Design review of the part built by this model. Coordinates are the model's own, in mm. Round coordinates to 2 decimals unless told otherwise and drop trailing zeros. Order: outer loops, then holes, each group sorted by start corner. A loop starts at its lowest first (then second) coordinate and runs counter-clockwise, first axis right, second up. Notation, with made-up numbers: (21.5, 3.5) - (50.5, 3.5) arc R26 cw to (50.5, 19.5) - close; hole circle Ø1 at (-17, 77.5). An arc over 180 degrees is marked (long way). Use CSV: the item, a comma, the result in double quotes.
from build123d import *

# Parameters (mm, degrees)
SKETCH1_W           = 63.2
SKETCH1_H           = 43.1
BOSS_EXTRUDE1_DEPTH = 1
CUT_EXTRUDE1_REACH  = 78.504
SKETCH2_R           = 1.25
CUT_EXTRUDE2_REACH  = 78.504
SKETCH3_R           = 0.4
CUT_EXTRUDE18_REACH = 78.504
SKETCH25_R          = 1.663368104


with BuildPart() as part:
    # Sketch1 → Boss-Extrude1 (new body)
    with BuildSketch(Plane(origin=(0, 0, 0), x_dir=(1, 0, 0), z_dir=(0, 1, 0))):
        with Locations((31.6, 21.55)):
            Rectangle(SKETCH1_W, SKETCH1_H)
    extrude(amount=BOSS_EXTRUDE1_DEPTH)

    # Sketch2 → Cut-Extrude1 (cut, up to next)
    with BuildSketch(Plane(origin=(0, 1, 0), x_dir=(1, 0, 0), z_dir=(0, 1, 0)), mode=Mode.PRIVATE) as cut_extrude1_sk1:
        with Locations(Location((3.5, 40.1, 0), (0, 0, 270))):
            Circle(SKETCH2_R)
    cut_extrude1_tool1 = extrude(cut_extrude1_sk1.sketch, amount=-CUT_EXTRUDE1_REACH, mode=Mode.PRIVATE) & part.part
    # Sketch2 → Cut-Extrude1 (cut, up to next)
    with BuildSketch(Plane(origin=(0, 1, 0), x_dir=(1, 0, 0), z_dir=(0, 1, 0)), mode=Mode.PRIVATE) as cut_extrude1_sk2:
        with Locations(Location((59.7, 40.1, 0), (0, 0, 270))):
            Circle(SKETCH2_R)
    cut_extrude1_tool2 = extrude(cut_extrude1_sk2.sketch, amount=-CUT_EXTRUDE1_REACH, mode=Mode.PRIVATE) & part.part
    # Sketch2 → Cut-Extrude1 (cut, up to next)
    with BuildSketch(Plane(origin=(0, 1, 0), x_dir=(1, 0, 0), z_dir=(0, 1, 0)), mode=Mode.PRIVATE) as cut_extrude1_sk3:
        with Locations(Location((59.7, 3, 0), (0, 0, 270))):
            Circle(SKETCH2_R)
    cut_extrude1_tool3 = extrude(cut_extrude1_sk3.sketch, amount=-CUT_EXTRUDE1_REACH, mode=Mode.PRIVATE) & part.part
    # Sketch2 → Cut-Extrude1 (cut, up to next)
    with BuildSketch(Plane(origin=(0, 1, 0), x_dir=(1, 0, 0), z_dir=(0, 1, 0)), mode=Mode.PRIVATE) as cut_extrude1_sk4:
        with Locations(Location((3.5, 3, 0), (0, 0, 270))):
            Circle(SKETCH2_R)
    cut_extrude1_tool4 = extrude(cut_extrude1_sk4.sketch, amount=-CUT_EXTRUDE1_REACH, mode=Mode.PRIVATE) & part.part
    add(cut_extrude1_tool1.solids().sort_by_distance((3.5, 1, -40.1))[0], mode=Mode.SUBTRACT)
    add(cut_extrude1_tool2.solids().sort_by_distance((59.7, 1, -40.1))[0], mode=Mode.SUBTRACT)
    add(cut_extrude1_tool3.solids().sort_by_distance((59.7, 1, -3))[0], mode=Mode.SUBTRACT)
    add(cut_extrude1_tool4.solids().sort_by_distance((3.5, 1, -3))[0], mode=Mode.SUBTRACT)

    # Sketch3 → Cut-Extrude2 (cut, up to next)
    with BuildSketch(Plane(origin=(0, 1, 0), x_dir=(1, 0, 0), z_dir=(0, 1, 0)), mode=Mode.PRIVATE) as cut_extrude2_sk1:
        with Locations(Location((7.47, 2.5, 0), (0, 0, 270))):
            Circle(SKETCH3_R)
    cut_extrude2_tool1 = extrude(cut_extrude2_sk1.sketch, amount=-CUT_EXTRUDE2_REACH, mode=Mode.PRIVATE) & part.part
    # Sketch3 → Cut-Extrude2 (cut, up to next)
    with BuildSketch(Plane(origin=(0, 1, 0), x_dir=(1, 0, 0), z_dir=(0, 1, 0)), mode=Mode.PRIVATE) as cut_extrude2_sk2:
        with Locations(Location((10.01, 2.5, 0), (0, 0, 270))):
            Circle(SKETCH3_R)
    cut_extrude2_tool2 = extrude(cut_extrude2_sk2.sketch, amount=-CUT_EXTRUDE2_REACH, mode=Mode.PRIVATE) & part.part
    # Sketch3 → Cut-Extrude2 (cut, up to next)
    with BuildSketch(Plane(origin=(0, 1, 0), x_dir=(1, 0, 0), z_dir=(0, 1, 0)), mode=Mode.PRIVATE) as cut_extrude2_sk3:
        with Locations(Location((12.55, 2.5, 0), (0, 0, 270))):
            Circle(SKETCH3_R)
    cut_extrude2_tool3 = extrude(cut_extrude2_sk3.sketch, amount=-CUT_EXTRUDE2_REACH, mode=Mode.PRIVATE) & part.part
    # Sketch3 → Cut-Extrude2 (cut, up to next)
    with BuildSketch(Plane(origin=(0, 1, 0), x_dir=(1, 0, 0), z_dir=(0, 1, 0)), mode=Mode.PRIVATE) as cut_extrude2_sk4:
        with Locations(Location((15.09, 2.5, 0), (0, 0, 270))):
            Circle(SKETCH3_R)
    cut_extrude2_tool4 = extrude(cut_extrude2_sk4.sketch, amount=-CUT_EXTRUDE2_REACH, mode=Mode.PRIVATE) & part.part
    # Sketch3 → Cut-Extrude2 (cut, up to next)
    with BuildSketch(Plane(origin=(0, 1, 0), x_dir=(1, 0, 0), z_dir=(0, 1, 0)), mode=Mode.PRIVATE) as cut_extrude2_sk5:
        with Locations(Location((17.63, 2.5, 0), (0, 0, 270))):
            Circle(SKETCH3_R)
    cut_extrude2_tool5 = extrude(cut_extrude2_sk5.sketch, amount=-CUT_EXTRUDE2_REACH, mode=Mode.PRIVATE) & part.part
    # Sketch3 → Cut-Extrude2 (cut, up to next)
    with BuildSketch(Plane(origin=(0, 1, 0), x_dir=(1, 0, 0), z_dir=(0, 1, 0)), mode=Mode.PRIVATE) as cut_extrude2_sk6:
        with Locations(Location((20.17, 2.5, 0), (0, 0, 270))):
            Circle(SKETCH3_R)
    cut_extrude2_tool6 = extrude(cut_extrude2_sk6.sketch, amount=-CUT_EXTRUDE2_REACH, mode=Mode.PRIVATE) & part.part
    # Sketch3 → Cut-Extrude2 (cut, up to next)
    with BuildSketch(Plane(origin=(0, 1, 0), x_dir=(1, 0, 0), z_dir=(0, 1, 0)), mode=Mode.PRIVATE) as cut_extrude2_sk7:
        with Locations(Location((22.71, 2.5, 0), (0, 0, 270))):
            Circle(SKETCH3_R)
    cut_extrude2_tool7 = extrude(cut_extrude2_sk7.sketch, amount=-CUT_EXTRUDE2_REACH, mode=Mode.PRIVATE) & part.part
    # Sketch3 → Cut-Extrude2 (cut, up to next)
    with BuildSketch(Plane(origin=(0, 1, 0), x_dir=(1, 0, 0), z_dir=(0, 1, 0)), mode=Mode.PRIVATE) as cut_extrude2_sk8:
        with Locations(Location((25.25, 2.5, 0), (0, 0, 270))):
            Circle(SKETCH3_R)
    cut_extrude2_tool8 = extrude(cut_extrude2_sk8.sketch, amount=-CUT_EXTRUDE2_REACH, mode=Mode.PRIVATE) & part.part
    # Sketch3 → Cut-Extrude2 (cut, up to next)
    with BuildSketch(Plane(origin=(0, 1, 0), x_dir=(1, 0, 0), z_dir=(0, 1, 0)), mode=Mode.PRIVATE) as cut_extrude2_sk9:
        with Locations(Location((27.79, 2.5, 0), (0, 0, 270))):
            Circle(SKETCH3_R)
    cut_extrude2_tool9 = extrude(cut_extrude2_sk9.sketch, amount=-CUT_EXTRUDE2_REACH, mode=Mode.PRIVATE) & part.part
    # Sketch3 → Cut-Extrude2 (cut, up to next)
    with BuildSketch(Plane(origin=(0, 1, 0), x_dir=(1, 0, 0), z_dir=(0, 1, 0)), mode=Mode.PRIVATE) as cut_extrude2_sk10:
        with Locations(Location((30.33, 2.5, 0), (0, 0, 270))):
            Circle(SKETCH3_R)
    cut_extrude2_tool10 = extrude(cut_extrude2_sk10.sketch, amount=-CUT_EXTRUDE2_REACH, mode=Mode.PRIVATE) & part.part
    # Sketch3 → Cut-Extrude2 (cut, up to next)
    with BuildSketch(Plane(origin=(0, 1, 0), x_dir=(1, 0, 0), z_dir=(0, 1, 0)), mode=Mode.PRIVATE) as cut_extrude2_sk11:
        with Locations(Location((32.87, 2.5, 0), (0, 0, 270))):
            Circle(SKETCH3_R)
    cut_extrude2_tool11 = extrude(cut_extrude2_sk11.sketch, amount=-CUT_EXTRUDE2_REACH, mode=Mode.PRIVATE) & part.part
    # Sketch3 → Cut-Extrude2 (cut, up to next)
    with BuildSketch(Plane(origin=(0, 1, 0), x_dir=(1, 0, 0), z_dir=(0, 1, 0)), mode=Mode.PRIVATE) as cut_extrude2_sk12:
        with Locations(Location((35.41, 2.5, 0), (0, 0, 270))):
            Circle(SKETCH3_R)
    cut_extrude2_tool12 = extrude(cut_extrude2_sk12.sketch, amount=-CUT_EXTRUDE2_REACH, mode=Mode.PRIVATE) & part.part
    # Sketch3 → Cut-Extrude2 (cut, up to next)
    with BuildSketch(Plane(origin=(0, 1, 0), x_dir=(1, 0, 0), z_dir=(0, 1, 0)), mode=Mode.PRIVATE) as cut_extrude2_sk13:
        with Locations(Location((37.95, 2.5, 0), (0, 0, 270))):
            Circle(SKETCH3_R)
    cut_extrude2_tool13 = extrude(cut_extrude2_sk13.sketch, amount=-CUT_EXTRUDE2_REACH, mode=Mode.PRIVATE) & part.part
    # Sketch3 → Cut-Extrude2 (cut, up to next)
    with BuildSketch(Plane(origin=(0, 1, 0), x_dir=(1, 0, 0), z_dir=(0, 1, 0)), mode=Mode.PRIVATE) as cut_extrude2_sk14:
        with Locations(Location((40.49, 2.5, 0), (0, 0, 270))):
            Circle(SKETCH3_R)
    cut_extrude2_tool14 = extrude(cut_extrude2_sk14.sketch, amount=-CUT_EXTRUDE2_REACH, mode=Mode.PRIVATE) & part.part
    # Sketch3 → Cut-Extrude2 (cut, up to next)
    with BuildSketch(Plane(origin=(0, 1, 0), x_dir=(1, 0, 0), z_dir=(0, 1, 0)), mode=Mode.PRIVATE) as cut_extrude2_sk15:
        with Locations(Location((43.03, 2.5, 0), (0, 0, 270))):
            Circle(SKETCH3_R)
    cut_extrude2_tool15 = extrude(cut_extrude2_sk15.sketch, amount=-CUT_EXTRUDE2_REACH, mode=Mode.PRIVATE) & part.part
    # Sketch3 → Cut-Extrude2 (cut, up to next)
    with BuildSketch(Plane(origin=(0, 1, 0), x_dir=(1, 0, 0), z_dir=(0, 1, 0)), mode=Mode.PRIVATE) as cut_extrude2_sk16:
        with Locations(Location((45.57, 2.5, 0), (0, 0, 270))):
            Circle(SKETCH3_R)
    cut_extrude2_tool16 = extrude(cut_extrude2_sk16.sketch, amount=-CUT_EXTRUDE2_REACH, mode=Mode.PRIVATE) & part.part
    # Sketch3 → Cut-Extrude2 (cut, up to next)
    with BuildSketch(Plane(origin=(0, 1, 0), x_dir=(1, 0, 0), z_dir=(0, 1, 0)), mode=Mode.PRIVATE) as cut_extrude2_sk17:
        with Locations(Location((48.11, 2.5, 0), (0, 0, 270))):
            Circle(SKETCH3_R)
    cut_extrude2_tool17 = extrude(cut_extrude2_sk17.sketch, amount=-CUT_EXTRUDE2_REACH, mode=Mode.PRIVATE) & part.part
    # Sketch3 → Cut-Extrude2 (cut, up to next)
    with BuildSketch(Plane(origin=(0, 1, 0), x_dir=(1, 0, 0), z_dir=(0, 1, 0)), mode=Mode.PRIVATE) as cut_extrude2_sk18:
        with Locations(Location((50.65, 2.5, 0), (0, 0, 270))):
            Circle(SKETCH3_R)
    cut_extrude2_tool18 = extrude(cut_extrude2_sk18.sketch, amount=-CUT_EXTRUDE2_REACH, mode=Mode.PRIVATE) & part.part
    # Sketch3 → Cut-Extrude2 (cut, up to next)
    with BuildSketch(Plane(origin=(0, 1, 0), x_dir=(1, 0, 0), z_dir=(0, 1, 0)), mode=Mode.PRIVATE) as cut_extrude2_sk19:
        with Locations(Location((53.19, 2.5, 0), (0, 0, 270))):
            Circle(SKETCH3_R)
    cut_extrude2_tool19 = extrude(cut_extrude2_sk19.sketch, amount=-CUT_EXTRUDE2_REACH, mode=Mode.PRIVATE) & part.part
    # Sketch3 → Cut-Extrude2 (cut, up to next)
    with BuildSketch(Plane(origin=(0, 1, 0), x_dir=(1, 0, 0), z_dir=(0, 1, 0)), mode=Mode.PRIVATE) as cut_extrude2_sk20:
        with Locations(Location((55.73, 2.5, 0), (0, 0, 270))):
            Circle(SKETCH3_R)
    cut_extrude2_tool20 = extrude(cut_extrude2_sk20.sketch, amount=-CUT_EXTRUDE2_REACH, mode=Mode.PRIVATE) & part.part
    add(cut_extrude2_tool1.solids().sort_by_distance((7.47, 1, -2.5))[0], mode=Mode.SUBTRACT)
    add(cut_extrude2_tool2.solids().sort_by_distance((10.01, 1, -2.5))[0], mode=Mode.SUBTRACT)
    add(cut_extrude2_tool3.solids().sort_by_distance((12.55, 1, -2.5))[0], mode=Mode.SUBTRACT)
    add(cut_extrude2_tool4.solids().sort_by_distance((15.09, 1, -2.5))[0], mode=Mode.SUBTRACT)
    add(cut_extrude2_tool5.solids().sort_by_distance((17.63, 1, -2.5))[0], mode=Mode.SUBTRACT)
    add(cut_extrude2_tool6.solids().sort_by_distance((20.17, 1, -2.5))[0], mode=Mode.SUBTRACT)
    add(cut_extrude2_tool7.solids().sort_by_distance((22.71, 1, -2.5))[0], mode=Mode.SUBTRACT)
    add(cut_extrude2_tool8.solids().sort_by_distance((25.25, 1, -2.5))[0], mode=Mode.SUBTRACT)
    add(cut_extrude2_tool9.solids().sort_by_distance((27.79, 1, -2.5))[0], mode=Mode.SUBTRACT)
    add(cut_extrude2_tool10.solids().sort_by_distance((30.33, 1, -2.5))[0], mode=Mode.SUBTRACT)
    add(cut_extrude2_tool11.solids().sort_by_distance((32.87, 1, -2.5))[0], mode=Mode.SUBTRACT)
    add(cut_extrude2_tool12.solids().sort_by_distance((35.41, 1, -2.5))[0], mode=Mode.SUBTRACT)
    add(cut_extrude2_tool13.solids().sort_by_distance((37.95, 1, -2.5))[0], mode=Mode.SUBTRACT)
    add(cut_extrude2_tool14.solids().sort_by_distance((40.49, 1, -2.5))[0], mode=Mode.SUBTRACT)
    add(cut_extrude2_tool15.solids().sort_by_distance((43.03, 1, -2.5))[0], mode=Mode.SUBTRACT)
    add(cut_extrude2_tool16.solids().sort_by_distance((45.57, 1, -2.5))[0], mode=Mode.SUBTRACT)
    add(cut_extrude2_tool17.solids().sort_by_distance((48.11, 1, -2.5))[0], mode=Mode.SUBTRACT)
    add(cut_extrude2_tool18.solids().sort_by_distance((50.65, 1, -2.5))[0], mode=Mode.SUBTRACT)
    add(cut_extrude2_tool19.solids().sort_by_distance((53.19, 1, -2.5))[0], mode=Mode.SUBTRACT)
    add(cut_extrude2_tool20.solids().sort_by_distance((55.73, 1, -2.5))[0], mode=Mode.SUBTRACT)

    # Sketch25 → Cut-Extrude18 (cut, up to next)
    with BuildSketch(Plane.XZ, mode=Mode.PRIVATE) as cut_extrude18_sk1:
        with Locations(Location((11.478536319, -7.136146005, 0), (0, 0, 270))):
            Circle(SKETCH25_R)
    cut_extrude18_tool1 = extrude(cut_extrude18_sk1.sketch, amount=-CUT_EXTRUDE18_REACH, mode=Mode.PRIVATE) & part.part
    add(cut_extrude18_tool1.solids().sort_by_distance((11.478536, 0, -7.136146))[0], mode=Mode.SUBTRACT)


solid = part.part
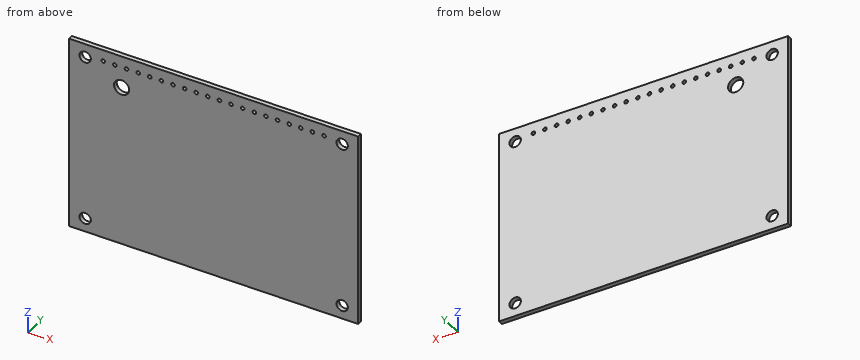
1) To check wall thickness, follow L1, parallel to X at y = 0.2, z = -3; L2, parallel to X at y = 0.55, z = -7; L3, parallel to Z at x = 35.41, y = 0.75. State the ranges of each line that lie inside material, in increasing order. Write a range as from..to.
Data:
L1,"x = 0..2.25, 4.75..58.45, 60.95..63.2"
L2,"x = 0..9.82, 13.14..63.2"
L3,"z = -43.1..-2.9, -2.1..0"
2) We need section B-B (z = -40.1). Give the boundary of the cut face in (x, y), then the cut area to 3 significant figures.
Data:
outline,"(0, 0) - (2.25, 0) - (2.25, 1) - (0, 1) - close; (4.75, 0) - (58.45, 0) - (58.45, 1) - (4.75, 1) - close; (60.95, 0) - (63.2, 0) - (63.2, 1) - (60.95, 1) - close"
area,"58.2 mm2"
3) Insertion check: pin 1 Ø4 at (x, z) = (59.7, -40.1) entering from -Y. The pin has a flat end and moves straight along its axis. Give the tip position at first contact, or say it passes through.
Data:
pin 1,"stops at y = 0"
4) We need section A-A (x = 3.5). Give the boundary of the cut face in (y, z), then the cut area to 3 significant figures.
Data:
outline,"(0, -43.1) - (1, -43.1) - (1, -41.35) - (0, -41.35) - close; (0, -38.85) - (1, -38.85) - (1, -4.25) - (0, -4.25) - close; (0, -1.75) - (1, -1.75) - (1, 0) - (0, 0) - close"
area,"38.1 mm2"
